Could you check a few things on this model? Use its own coordinates, in mm. Face numbers are marked on the shaded views. Round coordinates to 2 decimals unless told otherwise and drop trailing zeros. Loops run counter-clockwise (first coordinate to the right, second up) from the corner with the lowest first, then second, coordinate; pieces in that order, holes last. Notation, with made-up numbers: M 1.25,6 L 8.25,6 A19 ccw 8.25,12 Z; hole C 73,-32.75 d8. An arc over 180 degrees is marked long. Answer in a Markdown table with one row per item.
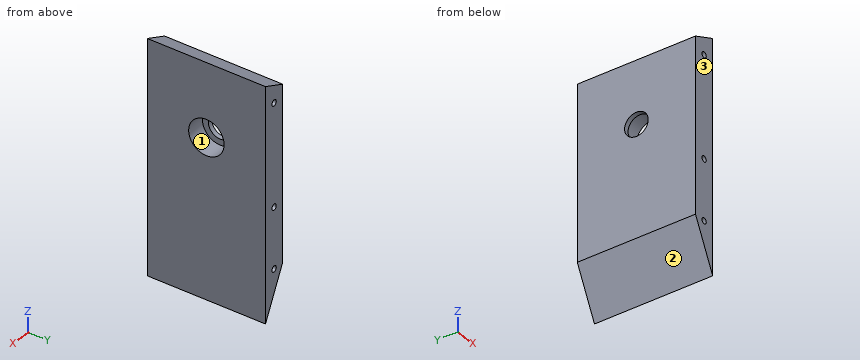
Autodesk Inventor part; units mm, degrees
ref_plane "Work Plane1" through (-5, 0, -36.75) normal (-1, 0, 0) x (0, 0, 1)
ref_plane "YZ Plane" through (0, 0, 0) normal (1, 0, 0) x (0, 1, 0)
ref_plane "XZ Plane" through (0, 0, 0) normal (0, 1, 0) x (-1, 0, 0)
sketch "Sketch1" plane through (0, 0, 0) normal (0, 1, 0) x (-1, 0, 0)
  line L0 (5, -36.75) -> (5, 36.75)
  line L1 (-5, 36.75) -> (-5, -36.75)
  line L2 (-5, 36.75) -> (-5, 41.1944)
  line L3 (5, 36.75) -> (-5, 41.1944)
  line L4 (-5, -36.75) -> (-5, -56.75)
  line L5 (-5, -56.75) -> (5, -36.75)
  line L6 (5, 11.25) -> (5, -36.75)
  line L7 (5, -31.75) -> (5, -36.75)
  line L8 (5, 31.75) -> (5, 36.75)
  circle A0 centre (0, 31.75) radius 1.25
  circle A1 centre (0, -36.75) radius 1.25
  circle A2 centre (0, -11.25) radius 1.25
  point P0 (0, 0)
  dimension "d3" = 10
  dimension "d4" = 73.5
  dimension "d6" = 4.4444
  dimension "d8" = 20
  dimension "d17" = 2.5
  dimension "d26" = 2.5
  dimension "d28" = 2.5
ref_plane "Work Plane1" through (-5, 0, -36.75) normal (-1, 0, 0) x (0, 0, 1)
extrude "Extrusion3" add sketch "Sketch1" along normal blind 50
sketch "Sketch3" plane through (-5, 0, -36.75) normal (-1, 0, 0) x (0, 0, 1)
  line L0 (73.5, 50) -> (47, 50)
  line L1 (47, 50) -> (47, 25)
  line L2 (47, 25) -> (73.5, 25)
  line L3 (73.5, 25) -> (73.5, 50)
  circle A0 centre (47, 25) radius 7.5
  circle A1 centre (47, 25) radius 5
  point P0 (36.75, 0)
  dimension "d37" = 26.5
  dimension "d38" = 25
  dimension "d39" = 15
  dimension "d42" = 10
extrude "Extrusion6" cut sketch "Sketch3" against normal blind 10 contours A0 L2 A1 L1 | L1 A1 L2 A0 | A1 L2 L1 | L1 L2 A1
extrude "Extrusion7" add sketch "Sketch3" against normal blind 2 contours A0 L2 A1 L1 | L1 A1 L2 A0
properties part number "bocnice_delsi"
1) I want a section at A-A, the plane z = 31.75. Please give me the cut outline in (x, y).
Computed:
| item | result |
|---|---|
| outline | M -5,0 L -1.25,0 L -1.25,50 L -5,50 Z; M 1.25,0 L 5,0 L 5,50 L 1.25,50 Z |
2) Will these pins go through, and if not, where does the flat tip stop? P1, Ø1.5, axis at x = -2.5, y = 44, coming from the +Z side; P2, Ø6, axis at x = -1.5, y = 11, coming from the +Z side; P3, Ø2, axis at x = 0, z = 31.75, coming from the -Y side; P4, Ø13, axis at y = 25, z = 10.25, coming from the +X side.
Computed:
| item | result |
|---|---|
| P1 | stops at z = 38.19 |
| P2 | stops at z = 39.64 |
| P3 | passes through |
| P4 | stops at x = -3 |
3) I want a section at C-C, the plane x = 0. Please give me the cut outline in (y, z), plus the area to 3 significant figures.
Computed:
| item | result |
|---|---|
| outline | M 0,-46.75 L 50,-46.75 L 50,-38 L 0,-38 Z; M 0,-35.5 L 50,-35.5 L 50,-12.5 L 0,-12.5 Z; M 0,-10 L 50,-10 L 50,30.5 L 0,30.5 Z; M 0,33 L 50,33 L 50,38.97 L 0,38.97 Z; hole C 25,10.25 d15 |
| area | 3,730 mm² |
4) If we mould it in two halves opening along Z, with no side actions, what happens to the marked faces 1, 2 and 3? For each: released by +Z, released by -Z, zero draft, split by the parting line, or undercut.
Computed:
| item | result |
|---|---|
| face 1 | undercut |
| face 2 | released by -Z |
| face 3 | zero draft |
5) I want a section at D-D, the plane y = 47. Please give me the cut outline in (x, z).
Computed:
| item | result |
|---|---|
| outline | M -5,-36.75 L 5,-56.75 L 5,41.19 L -5,36.75 Z; hole C 0,-36.75 d2.5; hole C 0,-11.25 d2.5; hole C 0,31.75 d2.5 |
6) I want a section at B-B, the plane y = 25. Please give me the cut outline in (x, z).
Computed:
| item | result |
|---|---|
| outline | M -5,-36.75 L 5,-56.75 L 5,2.75 L -3,2.75 L -3,5.25 L -5,5.25 Z; M -5,15.25 L -3,15.25 L -3,17.75 L 5,17.75 L 5,41.19 L -5,36.75 Z; hole C 0,-36.75 d2.5; hole C 0,-11.25 d2.5; hole C 0,31.75 d2.5 |
7) I need wall thicknesses on line 1 (Y direction, x = 1.5, z = 10.25); line 2 (Z direction, x = 0.75, y = 15); line 3 (Z direction, x = 0, y = 16.5). Which ranges of each line are inside material? Lowest first, please.
Computed:
| item | result |
|---|---|
| line 1 | y = 0 to 17.5, 32.5 to 50 |
| line 2 | z = -48.25 to -37.75, -35.75 to -12.25, -10.25 to 30.75, 32.75 to 39.31 |
| line 3 | z = -46.75 to -38, -35.5 to -12.5, -10 to 30.5, 33 to 38.97 |
